from build123d import *

# Parameters (mm, degrees)
SKETCH1_W           = 225.425
SKETCH1_H           = 50.8
BOSS_EXTRUDE1_DEPTH = 3.175
SKETCH2_W           = 30
SKETCH2_H           = 3.175
BOSS_EXTRUDE2_DEPTH = 3.175
SKETCH3_R           = 13.5
SKETCH3_R_2         = 16.5
CUT_EXTRUDE1_DEPTH  = 4.175
SKETCH4_W           = 3.175
SKETCH4_H           = 30
CUT_EXTRUDE2_DEPTH  = 10
SKETCH5_W           = 30
SKETCH5_H           = 3.175
CUT_EXTRUDE3_DEPTH  = 4.175
SKETCH6_W           = 3.175
SKETCH6_H           = 15
CUT_EXTRUDE4_DEPTH  = 4.175
SKETCH7_W           = 20
SKETCH7_H           = 4.111240443
CUT_EXTRUDE5_DEPTH  = 4.175
FILLET1_R           = 1


with BuildPart() as part:
    # Sketch1 → Boss-Extrude1 (new body)
    with BuildSketch(Plane.XY):
        Rectangle(SKETCH1_W, SKETCH1_H)
    extrude(amount=BOSS_EXTRUDE1_DEPTH)

    # Sketch2 → Boss-Extrude2 (add)
    with BuildSketch(Plane(origin=(0, 25.4, 0), x_dir=(1, 0, 0), z_dir=(0, 1, 0))):
        with Locations((67.7125, -1.5875)):
            Rectangle(SKETCH2_W, SKETCH2_H)
        with Locations((7.7125, -1.5875)):
            Rectangle(SKETCH2_W, SKETCH2_H)
        with Locations((-52.2875, -1.5875)):
            Rectangle(SKETCH2_W, SKETCH2_H)
    extrude(amount=BOSS_EXTRUDE2_DEPTH)

    # Sketch3 → Cut-Extrude1 (cut, through all)
    with BuildSketch(Plane.XY.offset(3.175)):
        with Locations((72.7125, 0)):
            Circle(SKETCH3_R)
        with Locations((-112.7125, 0)):
            Circle(SKETCH3_R_2)
    extrude(amount=-CUT_EXTRUDE1_DEPTH, mode=Mode.SUBTRACT)

    # Sketch4 → Cut-Extrude2 (cut)
    with BuildSketch(Plane.XY.offset(3.175)):
        with Locations((104.775, 0)):
            Rectangle(SKETCH4_W, SKETCH4_H)
    extrude(amount=-CUT_EXTRUDE2_DEPTH, mode=Mode.SUBTRACT)

    # Sketch5 → Cut-Extrude3 (cut, through all)
    with BuildSketch(Plane.XY.offset(3.175)):
        with Locations((-4.77, -19.8125)):
            Rectangle(SKETCH5_W, SKETCH5_H)
    extrude(amount=-CUT_EXTRUDE3_DEPTH, mode=Mode.SUBTRACT)

    # Sketch6 → Cut-Extrude4 (cut, through all)
    with BuildSketch(Plane.XY.offset(3.175)):
        with Locations((-38.7125, 0.9)):
            Rectangle(SKETCH6_W, SKETCH6_H)
        with Locations((36.5125, 0.9)):
            Rectangle(SKETCH6_W, SKETCH6_H)
    extrude(amount=-CUT_EXTRUDE4_DEPTH, mode=Mode.SUBTRACT)

    # Sketch7 → Cut-Extrude5 (cut, through all)
    with BuildSketch(Plane.XY.offset(3.175)):
        with Locations((74.6125, -23.344379779)):
            Rectangle(SKETCH7_W, SKETCH7_H)
    extrude(amount=-CUT_EXTRUDE5_DEPTH, mode=Mode.SUBTRACT)

    # Fillet1
    fillet1_edges = [part.edges().sort_by_distance(p)[0] for p in [
        (10.23, -18.225, 1.5875),
        (10.23, -21.4, 1.5875),
        (-19.77, -21.4, 1.5875),
        (-19.77, -18.225, 1.5875),
        (-37.125, 8.4, 1.5875),
        (-37.125, -6.6, 1.5875),
        (-40.3, -6.6, 1.5875),
        (-40.3, 8.4, 1.5875),
        (34.925, -6.6, 1.5875),
        (34.925, 8.4, 1.5875),
        (38.1, 8.4, 1.5875),
        (38.1, -6.6, 1.5875),
        (82.7125, 28.575, 1.5875),
        (52.7125, 28.575, 1.5875),
        (-7.2875, 28.575, 1.5875),
        (22.7125, 28.575, 1.5875),
        (-67.2875, 28.575, 1.5875),
        (-37.2875, 28.575, 1.5875),
        (103.1875, -15, 1.5875),
        (103.1875, 15, 1.5875),
        (106.3625, 15, 1.5875),
        (106.3625, -15, 1.5875),
    ]]
    fillet(fillet1_edges, radius=FILLET1_R)


solid = part.part
CAD build for the part. Positions are in the model's coordinates, mm. Coordinates: 2 decimals unless noted, no trailing zeros. Write each loop counter-clockwise with the first axis right and the second up, starting at its lowest first coordinate (ties: lowest second). Pieces come first, ordered by that corner, then holes. Notation, with made-up numbers: (77.25, 84) - (90.25, 84) arc R15 cw to (90.25, 111) - close; hole circle Ø2 at (-14.5, 25.5). An arc over 180 degrees is marked (long way). Use a Markdown table: item, result. Add a question column.
Item 1: Drill centre lines: L1, parallel to X at y = 26, z = 1.15; L2, parallel to Y at x = -11.5, z = 0.9 (3 decimals); L3, parallel to X at y = 12.5, z = 2.05. Where is each one in solid material? Low to high. Write a range as from..to.
Item 2: Band-saw the part on B-B, the plane x = 4. Give the cut face in (y, z) (3 decimals), and give its area (3 significant figures).
Item 3: Band-saw the part on C-C, the plane z = 0.7. Give the number of separate pieces and of enclosed holes in the cut face, and give its area (3 significant figures).
Item 4: Band-saw the part on D-D, the plane x = 90.5. Give the cut face in (y, z) (3 decimals), and give its area (3 significant figures).
Item 5: Band-saw the part on A-A, the plane y = 0. Give the cut face in (x, z) (1 decimal), and give its area (3 significant figures).
Item 6: Mould opens along X. For faces 1 (the face through (-96.216, -0.363, 1.61)), 2 (the face through (85.183, -5.171, 1.61)), 3 (the face through (-2, 2, 3.175)) say: pulls with the +X half, pulls with the -X half, needs draft (parallel to the pull), parting line crosses it, or undercut.
Item 7: Flat gauge pins, fed straight in: pin 1 (1.6 mm diameter, centred on y = 1.5, z = 1, fed in from -X); pin 2 (1 mm diameter, centred on x = -29.5, z = 1.5, fed in from +Y); pin 3 (1.7 mm diameter, centred on y = 26.5, z = 2, fed in from -X). Where does each tip first touch, or does it go through?
Numbers:
| question | item | result |
|---|---|---|
| 1 | L1 | -67.29..-37.29, -7.29..22.71, 52.71..82.71 |
| 1 | L2 | -25.4..-21.4, -18.225..25.4 |
| 1 | L3 | -101.94..67.61, 77.81..103.19, 106.36..112.71 |
| 2 | outline | (-25.4, 0) - (-21.4, 0) - (-21.4, 3.175) - (-25.4, 3.175) - close; (-18.225, 0) - (28.575, 0) - (28.575, 3.175) - (-18.225, 3.175) - close |
| 2 | area | 161 mm2 |
| 3 | separate pieces | 1 |
| 3 | enclosed holes | 5 |
| 3 | area | 10,400 mm2 |
| 4 | outline | (-25.4, 0) - (25.4, 0) - (25.4, 3.175) - (-25.4, 3.175) - close |
| 4 | area | 161 mm2 |
| 5 | outline | (-96.2, 0) - (-40.3, 0) - (-40.3, 3.2) - (-96.2, 3.2) - close; (-37.1, 0) - (34.9, 0) - (34.9, 3.2) - (-37.1, 3.2) - close; (38.1, 0) - (59.2, 0) - (59.2, 3.2) - (38.1, 3.2) - close; (86.2, 0) - (103.2, 0) - (103.2, 3.2) - (86.2, 3.2) - close; (106.4, 0) - (112.7, 0) - (112.7, 3.2) - (106.4, 3.2) - close |
| 5 | area | 547 mm2 |
| 6 | face 1 | pulls with the -X half |
| 6 | face 2 | undercut |
| 6 | face 3 | needs draft |
| 7 | pin 1 | x = -96.37 |
| 7 | pin 2 | y = 25.4 |
| 7 | pin 3 | x = -67.29 |
